Design review of the part built by this model. Coordinates are the model's own, in mm. A direction names the side the tool comes from. Give positions to 0.01 mm unless a question says otherwise; leave off trailing zeros. Order: outer loops, then holes, each group sorted by start corner. A loop starts at its lowest first (then second) coordinate and runs counter-clockwise, first axis right, second up.
Autodesk Inventor part; units mm, degrees
ref_plane "Work Plane2" through (0, 0, 5) normal (0, 0, -1) x (-1, 0, 0)
ref_plane "YZ Plane" through (0, 0, 0) normal (1, 0, 0) x (0, 1, 0)
ref_plane "XZ Plane" through (0, 0, 0) normal (0, 1, 0) x (-1, 0, 0)
sketch "Sketch1" plane through (0, 0, 0) normal (0, 0, 1) x (1, 0, 0)
  circle A0 centre (0, 0) radius 10.75
  circle A1 centre (0, 0) radius 2.25
  dimension "d0" = 21.5
  dimension "d1" = 4.5
extrude "Extrusion1" add sketch "Sketch1" along normal blind 19
sketch "Sketch2" plane through (0, 0, 19) normal (0, 0, 1) x (1, 0, 0)
  line L0 (7.5, 0) -> (3.75, -6.4952)
  line L1 (3.75, -6.4952) -> (-3.75, -6.4952)
  line L2 (-3.75, -6.4952) -> (-7.5, 0)
  line L3 (-7.5, 0) -> (-3.75, 6.4952)
  line L4 (-3.75, 6.4952) -> (3.75, 6.4952)
  line L5 (3.75, 6.4952) -> (7.5, 0)
  point P0 (0, 0)
  point P1 (0, 0)
  dimension "d4" = 15
extrude "Extrusion2" cut sketch "Sketch2" against normal blind 5
sketch "Sketch9" plane through (0, 0, 19) normal (0, 0, 1) x (1, 0, 0)
  circle A0 centre (0, -6.35) radius 1.5
  circle A1 centre (0, 6.35) radius 1.5
  line L0 (0, 6.35) -> (0, -6.35) construction
  circle A2 centre (6.35, 0) radius 1.5
  circle A3 centre (-6.35, 0) radius 1.5
  line L1 (-6.35, 0) -> (6.35, 0) construction
  point P0 (0, 0)
  point P1 (0, 0)
  dimension "d19" = 3
  dimension "d20" = 3
  dimension "d21" = 12.7
  dimension "d22" = 3
  dimension "d23" = 3
  dimension "d24" = 12.7
extrude "Extrusion6" cut sketch "Sketch9" against normal through all
ref_plane "Work Plane2" through (0, 0, 5) normal (0, 0, -1) x (-1, 0, 0)
sketch "Sketch11" plane through (0, 0, 5) normal (0, 0, -1) x (-1, 0, 0)
  circle A0 centre (-6.35, 0) radius 1.5
  circle A1 centre (-6.35, 0) radius 3
  circle A2 centre (0, 0) radius 2.25 construction
  circle A3 centre (0, -6.35) radius 3
  circle A4 centre (6.35, 0) radius 3
  circle A5 centre (0, 6.35) radius 3
  point P0 (6.35, 0)
  point P1 (0, 6.35)
  point P2 (0, -6.35)
  dimension "d32" = 6
  dimension "d40" = 360
extrude "Extrusion7" cut sketch "Sketch11" against normal through all contours A0 | A1 | A3 | A4 | A5
properties part number "AA031" material "ABS Plastic"
1. Take a section at A-A (z = 17). State the section outline as (x, y) points.
Recorded:
outline: circle Ø21.5 at (0, 0); hole (-5.8, -2.95) - (-3.75, -6.5) - (-3, -6.5) arc R3 ccw to (3, -6.5) - (3.75, -6.5) - (5.8, -2.95) arc R3 ccw (long way) to (5.8, 2.95) - (3.75, 6.5) - (3, 6.5) arc R3 ccw to (-3, 6.5) - (-3.75, 6.5) - (-5.8, 2.95) arc R3 ccw (long way) to start
2. Take a section at D-D (z = 3.75). State the section outline as (x, y) points, then the cut area to 3 significant figures.
Recorded:
outline: circle Ø21.5 at (0, 0); hole circle Ø3 at (-6.35, 0); hole circle Ø4.5 at (0, 0); hole circle Ø3 at (0, -6.35); hole circle Ø3 at (0, 6.35); hole circle Ø3 at (6.35, 0)
area: 319 mm2
3. Draft analysis for pull direction Y (two halves, no side actions). For faces 3 (the face through (-1.4, -10.66, 9.37)), 4 (the face through (-5, -5, 19)), 5 (the face through (2.5, 0.1, 14)), state which applies: pulls with the +Y half, pulls with the -Y half, needs draft (parallel to the pull), parting line crosses it, or undercut.
Recorded:
face 3: parting line crosses it
face 4: needs draft
face 5: undercut
4. Machinability: for faces 1 (the face through (8, -1, 5)), 2 (the face through (-4.964, -0.575, 2.535)), which of the approach directions +Z, -Z, +X, -X, +Y, -Y give a long, thin tool a straight path to every point of the face, cutting with its end or side? Answer none if there is none.
Recorded:
face 1: +Z
face 2: +Z, -Z
5. For pin 1 (3.5 mm diameter, centred on x = 1, y = 2.5, fed in from +Z); pin 2 (5 mm diameter, centred on x = 5, z = 13.5, fed in from +Y); pin 3 (3.5 mm diameter, centred on x = 0, y = 6.35, fed in from +Z), all flat-tipped, find the tip position at first contact; note any pin that passes through.
Recorded:
pin 1: stops at z = 14
pin 2: stops at y = 10.46
pin 3: stops at z = 5
6. For line 1 along Y through (x, z) = (0, 10); line 2 along Y through (x, z) = (0, 3.7); line 3 along X through (y, z) = (-2.75, 8), list the stretches that pass through material, from the lowest coordinate up.
Recorded:
line 1: y = -10.75 to -9.35, -3.35 to -2.25, 2.25 to 3.35, 9.35 to 10.75
line 2: y = -10.75 to -7.85, -4.85 to -2.25, 2.25 to 4.85, 7.85 to 10.75
line 3: x = -10.39 to -7.55, -5.15 to 5.15, 7.55 to 10.39
7. Take a section at C-C (y = 0). State the section outline as (x, z) points, then the cut area to 3 significant figures.
Recorded:
outline: (-10.75, 0) - (-7.85, 0) - (-7.85, 5) - (-9.35, 5) - (-9.35, 19) - (-10.75, 19) - close; (-4.85, 0) - (-2.25, 0) - (-2.25, 14) - (-3.35, 14) - (-3.35, 5) - (-4.85, 5) - close; (2.25, 0) - (4.85, 0) - (4.85, 5) - (3.35, 5) - (3.35, 14) - (2.25, 14) - close; (7.85, 0) - (10.75, 0) - (10.75, 19) - (9.35, 19) - (9.35, 5) - (7.85, 5) - close
area: 114 mm2
8. Take a section at B-B (x = -6.35). State the section outline as (y, z) points, then the cut area to 3 significant figures.
Recorded:
outline: (-8.67, 0) - (-1.5, 0) - (-1.5, 5) - (-3, 5) - (-3, 19) - (-8.67, 19) - close; (1.5, 0) - (8.67, 0) - (8.67, 19) - (3, 19) - (3, 5) - (1.5, 5) - close
area: 231 mm2
